Could you check a few things on this drawing? It's one solid part, dimensions in mm from its lowest x, y, z. A direction names the side the tool comes from. Give positions to 0.01 mm unless a question says otherwise; leave off trailing zeros. Order: outer loops, then holes, each group sorted by start corner. A loop starts at its lowest first (then second) coordinate and runs counter-clockwise, first axis right, second up.
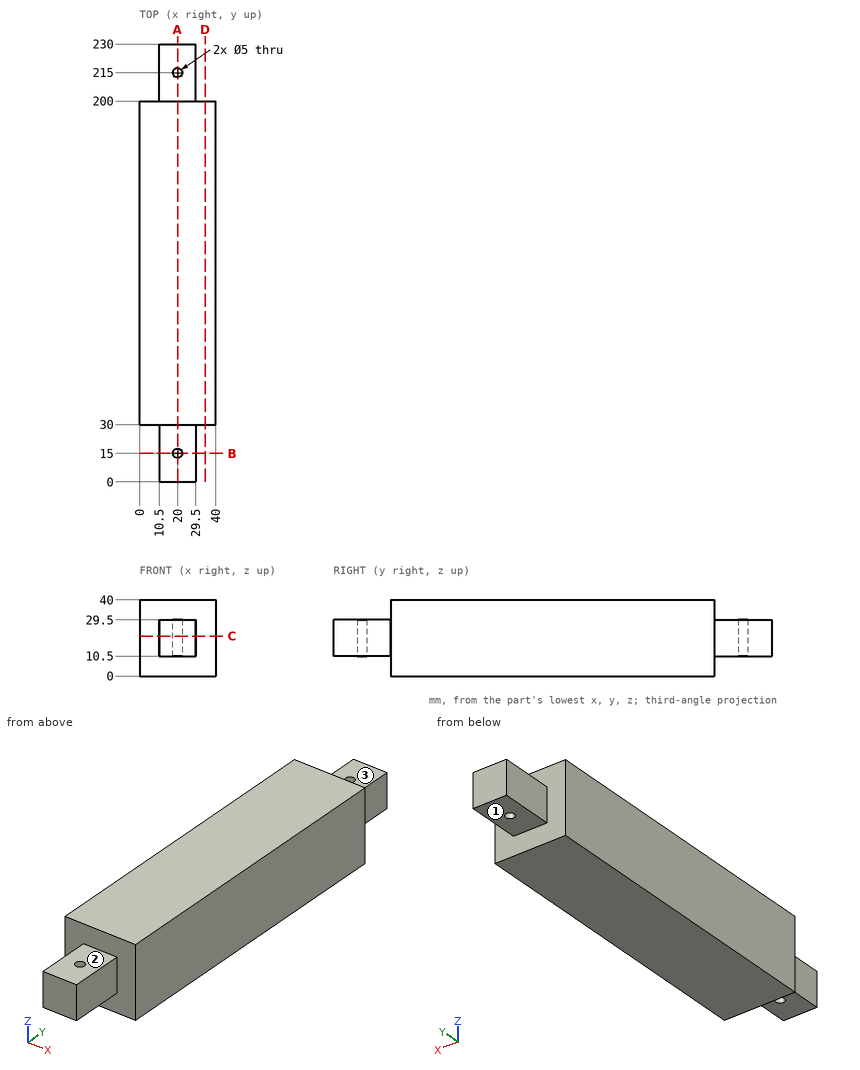
1) Suppose I cut it at A-A (x = 20). Please give me the cut outline in (y, z).
2) Suppose I cut it at B-B (y = 15). Please give me the cut outline in (x, z), and give its area (3 significant figures).
3) I'm going to push flat-ended pins straight in: pin 1 Ø15 at (x, y) = (15.5, 14.5) entering from -Z; pin 2 Ø2 at (x, z) = (7.5, 10) entering from -Y; pin 3 Ø9.5 at (x, y) = (19.5, 214) entering from +Z. Where does each tip first touch, or does it pass through?
4) Suppose I cut it at D-D (x = 34.5). Please give me the cut outline in (y, z), and give its area (3 significant figures).
5) Which directions (+Z, -Z, +X, -X, +Y, -Y) give clear straight access to the entire face, cutting with the end or side of a thin tool? Please do the marked faces 1, 2 and 3.
6) If I drill on line 1 (Y direction, x = 20, z = 21); line 2 (X direction, y = 215, z = 24.25); line 3 (Y direction, x = 2.5, z = 32.5), over which ranges is the centre line in solid material (lowest first)?
7) Suppose I cut it at C-C (z = 21). Please give me the cut outline in (x, y).
Results:
1. outline: (0, 10.5) - (12.5, 10.5) - (12.5, 29.5) - (0, 29.5) - close; (17.5, 10.5) - (30, 10.5) - (30, 0) - (200, 0) - (200, 10.5) - (212.5, 10.5) - (212.5, 29.5) - (200, 29.5) - (200, 40) - (30, 40) - (30, 29.5) - (17.5, 29.5) - close; (217.5, 10.5) - (230, 10.5) - (230, 29.5) - (217.5, 29.5) - close
2. outline: (10.5, 10.5) - (17.5, 10.5) - (17.5, 29.5) - (10.5, 29.5) - close; (22.5, 10.5) - (29.5, 10.5) - (29.5, 29.5) - (22.5, 29.5) - close
2. area: 266 mm2
3. pin 1: stops at z = 10.5
3. pin 2: stops at y = 30
3. pin 3: stops at z = 29.5
4. outline: (30, 0) - (200, 0) - (200, 40) - (30, 40) - close
4. area: 6,800 mm2
5. face 1: -Z, +X, -X, +Y
5. face 2: +Z, +X, -X, -Y
5. face 3: +Z, +X, -X, +Y
6. line 1: y = 0 to 12.5, 17.5 to 212.5, 217.5 to 230
6. line 2: x = 10.5 to 17.5, 22.5 to 29.5
6. line 3: y = 30 to 200
7. outline: (0, 30) - (10.5, 30) - (10.5, 0) - (29.5, 0) - (29.5, 30) - (40, 30) - (40, 200) - (29.5, 200) - (29.5, 230) - (10.5, 230) - (10.5, 200) - (0, 200) - close; hole circle Ø5 at (20, 15); hole circle Ø5 at (20, 215)
